Read the model definition and answer for the solid it produces. Units are mm, in the model's axes. A direction names the side the tool comes from. Round coordinates to 2 decimals unless told otherwise and drop trailing zeros. Order: outer loops, then holes, each group sorted by start corner. A loop starts at its lowest first (then second) coordinate and runs counter-clockwise, first axis right, second up. Notation, with made-up numbers: (-5.75, 12.5) -> (42.25, 12.5) arc R18 cw to (42.25, 43.5) -> close; hole circle Ø1 at (53.5, 11). An arc over 180 degrees is marked (long way). One line per item, written item: value. Start each with the question number.
1. Consider line 1 (X direction, y = -0.5, z = -4); line 2 (Y direction, x = 31.5, z = -31); line 3 (Z direction, x = 7, y = -6.5). Determine where each line is inside the solid, lowest interval first.
2. Flat-ended cylindrical pins translate along their axes: pin 1 Ø2 at (x, z) = (4.5, 17.5) entering from +Y; pin 2 Ø6.5 at (x, y) = (-1, 1) entering from -Z; pin 3 Ø10.5 at (y, z) = (-4, 4.5) entering from +X; pin 4 Ø12 at (x, z) = (5.5, 3) entering from +Y. Find the tip coordinate at first contact, or state that the pin passes through.
3. Section A-A (z = 13) is taken. Give the vertices of the cut face in (x, y), then the cut area to 3 significant figures.
4. Section B-B (y = 6.25) is taken. Give the vertices of the cut face in (x, z), then the cut area to 3 significant figures.
5. Section C-C (x = 15) is taken. Give the vertices of the cut face in (y, z).
6. For faces 1 (the face through (0, -3, -16.3)), 2 (the face through (8, 8, 0)), 3 (the face through (50, -17, -1)), 4 (the face through (3.5, 1, 14)), 5 (the face through (-6.45, 0, 0)), determine the directions among +Z, -Z, +X, -X, +Y, -Y from which every point of the face is accessible in a straight line to the end or side of a thin tool.
7. The mould has two halves that part along X. Classify faces 6 (the face through (11.45, -2, 0)), 7 (the face through (-45, -17, -45)), 8 (the face through (0, -6, 14)): released by +X, released by -X, zero draft, split by the parting line, or undercut.
8. Section D-D (y = -16.5) is taken. Give the vertices of the cut face in (x, z).
from build123d import *

# Parameters (mm, degrees)
SKETCH1_W               = 22.6
SKETCH1_H               = 16
BASE_BLOCK_DEPTH        = 6.45
SHELL1_T                = 5
CABLE_PASSTHROUGH_REACH = 25.786
SKETCH2_W               = 7
SKETCH2_H               = 14
SKETCH3_W               = 100
SKETCH3_H               = 100
BASE_PLATE_DEPTH        = 8
CORNER_CHAMFER_SIZE     = 10


with BuildPart() as part:
    # Sketch1 → base block (new, symmetric)
    with BuildSketch(Plane(origin=(0, 0, 0), x_dir=(0, 0, -1), z_dir=(1, 0, 0))):
        Rectangle(SKETCH1_W, SKETCH1_H)
    extrude(amount=BASE_BLOCK_DEPTH, both=True)

    # Shell1
    shell1_openings = [part.faces().sort_by_distance(p)[0] for p in [
        (0, 8, 0),
    ]]
    offset(amount=SHELL1_T, openings=shell1_openings, kind=Kind.INTERSECTION)

    # Sketch2 → cable passthrough (cut, up to next)
    with BuildSketch(Plane.XY, mode=Mode.PRIVATE) as cable_passthrough_sk1:
        with Locations((0, 1)):
            Rectangle(SKETCH2_W, SKETCH2_H)
    cable_passthrough_tool1 = extrude(cable_passthrough_sk1.sketch, amount=CABLE_PASSTHROUGH_REACH, mode=Mode.PRIVATE) & part.part
    add(cable_passthrough_tool1.solids().sort_by_distance((0, 1, 0))[0], mode=Mode.SUBTRACT)

    # Sketch3 → base plate (add)
    with BuildSketch(Plane.XZ.offset(13)):
        Rectangle(SKETCH3_W, SKETCH3_H)
    extrude(amount=BASE_PLATE_DEPTH)

    # corner chamfer
    corner_chamfer_edges = [part.edges().sort_by_distance(p)[0] for p in [
        (50, -17, -50),
        (50, -17, 50),
        (-50, -17, 50),
        (-50, -17, -50),
    ]]
    chamfer(corner_chamfer_edges, length=CORNER_CHAMFER_SIZE)


solid = part.part
Answer:
1. line 1: -11.45 to -6.45, 6.45 to 11.45
1. line 2: -21 to -13
1. line 3: -16.3 to 16.3
2. pin 1: y = -13
2. pin 2: z = -16.3
2. pin 3: x = 11.45
2. pin 4: y = 8
3. outline: (-50, -21) -> (50, -21) -> (50, -13) -> (11.45, -13) -> (11.45, 8) -> (3.5, 8) -> (3.5, -6) -> (-3.5, -6) -> (-3.5, 8) -> (-11.45, 8) -> (-11.45, -13) -> (-50, -13) -> close
3. area: 1,180 mm^2
4. outline: (-11.45, -16.3) -> (11.45, -16.3) -> (11.45, 16.3) -> (3.5, 16.3) -> (3.5, 11.3) -> (6.45, 11.3) -> (6.45, -11.3) -> (-6.45, -11.3) -> (-6.45, 11.3) -> (-3.5, 11.3) -> (-3.5, 16.3) -> (-11.45, 16.3) -> close
4. area: 420 mm^2
5. outline: (-21, -50) -> (-13, -50) -> (-13, 50) -> (-21, 50) -> close
6. face 1: -Z, +X, -X, +Y
6. face 2: +Z, -Z, +X, -X, +Y
6. face 3: +Z, -Z, +X, +Y, -Y
6. face 4: +Z, +Y
6. face 5: +Y
7. face 6: released by +X
7. face 7: released by -X
7. face 8: undercut
8. outline: (-50, -40) -> (-40, -50) -> (40, -50) -> (50, -40) -> (50, 40) -> (40, 50) -> (-40, 50) -> (-50, 40) -> close
